from build123d import *

# Parameters (mm, degrees)
BOSS_EXTRUDE1_DEPTH     = 52
SHELL1_START            = 3
SHELL1_DEPTH            = 46
SKETCH2_R               = 4.5
BOSS_EXTRUDE2_DEPTH     = 52
SKETCH3_R               = 3.25
CUT_EXTRUDE1_DEPTH      = 49
SKETCH4_R               = 1.7
CUT_EXTRUDE2_DEPTH      = 91.166512631
CUT_EXTRUDE3_DEPTH      = 20
CUT_EXTRUDE3_DEPTH_BACK = 20
CUT_EXTRUDE4_DEPTH      = 3.5
SKETCH7_R               = 4
CUT_EXTRUDE5_DEPTH      = 3.5
SKETCH8_W               = 6
SKETCH8_H               = 37
BOSS_EXTRUDE3_DEPTH     = 8
SKETCH9_W               = 1.9
SKETCH9_H               = 33.6
CUT_EXTRUDE6_DEPTH      = 6
SKETCH10_R              = 3
BOSS_EXTRUDE4_DEPTH     = 8


# Read off the part's stored shape, not the designer's step: Shell1
with BuildPart() as part:
    # Sketch1 → Boss-Extrude1 (new body)
    with BuildSketch(Plane.XY):
        with BuildLine():
            Line((-45, -55), (45, -55))
            ThreePointArc((45, -55), (52.071067812, -52.071067812), (55, -45))
            Line((55, -45), (55, -10))
            ThreePointArc((55, -10), (52.071067812, -2.928932188), (45, 0))
            Line((45, 0), (-45, 0))
            ThreePointArc((-45, 0), (-52.071067812, -2.928932188), (-55, -10))
            Line((-55, -10), (-55, -45))
            ThreePointArc((-55, -45), (-52.071067812, -52.071067812), (-45, -55))
        make_face()
    extrude(amount=BOSS_EXTRUDE1_DEPTH)

    # Shell1 outline → Shell1 (cut)
    with BuildSketch(Plane.XY.offset(SHELL1_START)):
        with BuildLine():
            Line((45, -3), (45, 0))
            Line((45, 0), (-45, 0))
            Line((-45, 0), (-45, -3))
            ThreePointArc((-45, -3), (-49.949747468, -5.050252532), (-52, -10))
            Line((-52, -10), (-52, -45))
            ThreePointArc((-52, -45), (-49.949747468, -49.949747468), (-45, -52))
            Line((-45, -52), (45, -52))
            ThreePointArc((45, -52), (49.949747468, -49.949747468), (52, -45))
            Line((52, -45), (52, -10))
            ThreePointArc((52, -10), (49.949747468, -5.050252532), (45, -3))
        make_face()
    extrude(amount=SHELL1_DEPTH, mode=Mode.SUBTRACT)

    # Sketch2 → Boss-Extrude2 (add)
    with BuildSketch(Plane(origin=(0, 0, 0), x_dir=(1, 0, 0), z_dir=(0, 1, 0))):
        with Locations(Location((-40, -8, 0), (0, 0, 270))):
            Circle(SKETCH2_R)
        with Locations(Location((40, -8, 0), (0, 0, 270))):
            Circle(SKETCH2_R)
        with Locations(Location((-40, -40, 0), (0, 0, 270))):
            Circle(SKETCH2_R)
        with Locations(Location((40, -40, 0), (0, 0, 270))):
            Circle(SKETCH2_R)
    extrude(amount=-BOSS_EXTRUDE2_DEPTH)

    # Sketch3 → Cut-Extrude1 (cut)
    with BuildSketch(Plane.XZ.offset(55)):
        with Locations(Location((-40, 8, 0), (0, 0, 270))):
            Circle(SKETCH3_R)
        with Locations(Location((40, 8, 0), (0, 0, 270))):
            Circle(SKETCH3_R)
        with Locations(Location((-40, 40, 0), (0, 0, 270))):
            Circle(SKETCH3_R)
        with Locations(Location((40, 40, 0), (0, 0, 270))):
            Circle(SKETCH3_R)
    extrude(amount=-CUT_EXTRUDE1_DEPTH, mode=Mode.SUBTRACT)

    # Sketch4 → Cut-Extrude2 (cut, through all)
    with BuildSketch(Plane.XZ.offset(6)):
        with Locations(Location((-40, 8, 0), (0, 0, 270))):
            Circle(SKETCH4_R)
        with Locations(Location((40, 8, 0), (0, 0, 270))):
            Circle(SKETCH4_R)
        with Locations(Location((-40, 40, 0), (0, 0, 270))):
            Circle(SKETCH4_R)
        with Locations(Location((40, 40, 0), (0, 0, 270))):
            Circle(SKETCH4_R)
    extrude(amount=-CUT_EXTRUDE2_DEPTH, mode=Mode.SUBTRACT)

    # Sketch5 → Cut-Extrude3 (cut, two sides: drawn at the far end of the back side and taken through both)
    with BuildSketch(Plane.XY.offset(26).offset(-CUT_EXTRUDE3_DEPTH_BACK)):
        Polygon((-51, -14), (-51, -11.5), (-55.5, -16), (-55.5, -18.5), align=None)
        Polygon((51, -14), (51, -11.5), (55.5, -16), (55.5, -18.5), align=None)
        Polygon((-51, -20), (-51, -17.5), (-55.5, -22), (-55.5, -24.5), align=None)
        Polygon((51, -20), (51, -17.5), (55.5, -22), (55.5, -24.5), align=None)
        Polygon((-51, -26), (-51, -23.5), (-55.5, -28), (-55.5, -30.5), align=None)
        Polygon((51, -26), (51, -23.5), (55.5, -28), (55.5, -30.5), align=None)
        Polygon((-51, -32), (-51, -29.5), (-55.5, -34), (-55.5, -36.5), align=None)
        Polygon((51, -32), (51, -29.5), (55.5, -34), (55.5, -36.5), align=None)
        Polygon((-51, -38), (-51, -35.5), (-55.5, -40), (-55.5, -42.5), align=None)
        Polygon((51, -38), (51, -35.5), (55.5, -40), (55.5, -42.5), align=None)
    extrude(amount=CUT_EXTRUDE3_DEPTH + CUT_EXTRUDE3_DEPTH_BACK, mode=Mode.SUBTRACT)

    # Sketch6 → Cut-Extrude4 (cut)
    with BuildSketch(Plane.XZ.offset(55)):
        with BuildLine():
            Line((-34.5, 12), (-34.5, 40))
            ThreePointArc((-34.5, 40), (-33, 41.5), (-31.5, 40))
            Line((-31.5, 40), (-31.5, 12))
            ThreePointArc((-31.5, 12), (-33, 10.5), (-34.5, 12))
        make_face()
        with BuildLine():
            Line((-28.5, 12), (-28.5, 40))
            ThreePointArc((-28.5, 40), (-27, 41.5), (-25.5, 40))
            Line((-25.5, 40), (-25.5, 12))
            ThreePointArc((-25.5, 12), (-27, 10.5), (-28.5, 12))
        make_face()
        with BuildLine():
            Line((-22.5, 12), (-22.5, 40))
            ThreePointArc((-22.5, 40), (-21, 41.5), (-19.5, 40))
            Line((-19.5, 40), (-19.5, 12))
            ThreePointArc((-19.5, 12), (-21, 10.5), (-22.5, 12))
        make_face()
        with BuildLine():
            Line((-16.5, 12), (-16.5, 40))
            ThreePointArc((-16.5, 40), (-15, 41.5), (-13.5, 40))
            Line((-13.5, 40), (-13.5, 12))
            ThreePointArc((-13.5, 12), (-15, 10.5), (-16.5, 12))
        make_face()
        with BuildLine():
            Line((-10.5, 12), (-10.5, 40))
            ThreePointArc((-10.5, 40), (-9, 41.5), (-7.5, 40))
            Line((-7.5, 40), (-7.5, 12))
            ThreePointArc((-7.5, 12), (-9, 10.5), (-10.5, 12))
        make_face()
        with BuildLine():
            Line((-4.5, 12), (-4.5, 40))
            ThreePointArc((-4.5, 40), (-3, 41.5), (-1.5, 40))
            Line((-1.5, 40), (-1.5, 12))
            ThreePointArc((-1.5, 12), (-3, 10.5), (-4.5, 12))
        make_face()
        with BuildLine():
            Line((1.5, 12), (1.5, 40))
            ThreePointArc((1.5, 40), (3, 41.5), (4.5, 40))
            Line((4.5, 40), (4.5, 12))
            ThreePointArc((4.5, 12), (3, 10.5), (1.5, 12))
        make_face()
        with BuildLine():
            Line((7.5, 12), (7.5, 40))
            ThreePointArc((7.5, 40), (9, 41.5), (10.5, 40))
            Line((10.5, 40), (10.5, 12))
            ThreePointArc((10.5, 12), (9, 10.5), (7.5, 12))
        make_face()
        with BuildLine():
            Line((13.5, 12), (13.5, 40))
            ThreePointArc((13.5, 40), (15, 41.5), (16.5, 40))
            Line((16.5, 40), (16.5, 12))
            ThreePointArc((16.5, 12), (15, 10.5), (13.5, 12))
        make_face()
        with BuildLine():
            Line((19.5, 12), (19.5, 40))
            ThreePointArc((19.5, 40), (21, 41.5), (22.5, 40))
            Line((22.5, 40), (22.5, 12))
            ThreePointArc((22.5, 12), (21, 10.5), (19.5, 12))
        make_face()
    extrude(amount=-CUT_EXTRUDE4_DEPTH, mode=Mode.SUBTRACT)

    # Sketch7 → Cut-Extrude5 (cut)
    with BuildSketch(Plane(origin=(0, 0, 0), x_dir=(-1, 0, 0), z_dir=(0, 0, -1))):
        with Locations((30, -12)):
            Circle(SKETCH7_R)
        with Locations((-30, -12)):
            Circle(SKETCH7_R)
    extrude(amount=-CUT_EXTRUDE5_DEPTH, mode=Mode.SUBTRACT)

    # Sketch8 → Boss-Extrude3 (add)
    with BuildSketch(Plane(origin=(0, -52, 0), x_dir=(1, 0, 0), z_dir=(0, 1, 0))):
        with Locations((30, -26)):
            Rectangle(SKETCH8_W, SKETCH8_H)
    extrude(amount=BOSS_EXTRUDE3_DEPTH)

    # Sketch9 → Cut-Extrude6 (cut)
    with BuildSketch(Plane(origin=(0, -44, 0), x_dir=(1, 0, 0), z_dir=(0, 1, 0))):
        with Locations((30, -26)):
            Rectangle(SKETCH9_W, SKETCH9_H)
    extrude(amount=-CUT_EXTRUDE6_DEPTH, mode=Mode.SUBTRACT)

    # Sketch10 → Boss-Extrude4 (add)
    with BuildSketch(Plane(origin=(0, -52, 0), x_dir=(1, 0, 0), z_dir=(0, 1, 0))):
        with Locations(Location((-29, -13, 0), (0, 0, 55.426050329))):
            Circle(SKETCH10_R)
        with Locations(Location((-29, -39, 0), (0, 0, 80.405931773))):
            Circle(SKETCH10_R)
        with Locations(Location((13, -13, 0), (0, 0, 55.426050329))):
            Circle(SKETCH10_R)
        with Locations(Location((13, -39, 0), (0, 0, 80.405931773))):
            Circle(SKETCH10_R)
    extrude(amount=BOSS_EXTRUDE4_DEPTH)


solid = part.part
CAD build for the part. Positions are in the model's coordinates, mm. A direction names the side the tool comes from. Coordinates: 2 decimals unless noted, no trailing zeros. Write each loop counter-clockwise with the first axis right and the second up, starting at its lowest first coordinate (ties: lowest second). Pieces come first, ordered by that corner, then holes. Notation, with made-up numbers: (-19.75, 44) - (31.25, 44) arc R25 ccw to (31.25, 58) - close; hole circle Ø5 at (-26, -20). An arc over 180 degrees is marked (long way). Use a Markdown table: item, result. Add a question column.
Item 1: Band-saw the part on A-A, the plane x = -15. Give the cut face in (y, z).
Item 2: Band-saw the part on B-B, the plane z = 31.5. Give the number of separate pieces and of enclosed holes in the cut face, and give its area (3 significant figures).
Item 3: 3-axis set-ups, long thin cutter, end or side, ignore diameter. For faces 1 (the face through (13, -44, 13)), 2 (the face through (-53.5, -38, 25.7)), 3 (the face through (-27, -53.5, 10.5)): which of +Z, -Z, +X, -X, +Y, -Y reach the whole face in a straight line?
Item 4: Flat gauge pins, fed straight in: pin 1 (7 mm diameter, centred on x = -39, z = 9, fed in from -Y); pin 2 (1.5 mm diameter, centred on y = -53.5, z = 31.5, fed in from +X); pin 3 (1.8 mm diameter, centred on x = -28.5, z = 38, fed in from +Y); pin 4 (1 mm diameter, centred on x = 32.5, y = -12, fed in from -Z). Where does each tip first touch, or does it go through?
Item 5: Drill centre lines: L1, parallel to Z at x = -4, y = -39; L2, parallel to Z at x = -38, y = -22; L3, parallel to X at y = -31.5, z = 40. Where is each one in solid material? Low to high. Write a range as from..to.
Item 6: Mould opens along X. For faces 4 (the face through (51.99, -52.15, 25.64)), 5 (the face through (33, -48, 26)), 6 (the face through (1, 0, 50)) say: pulls with the +X half, pulls with the -X half, needs draft (parallel to the pull), parting line crosses it, or undercut.
Item 7: Band-saw the part on C-C, the plane x = 47.5. Give the cut face in (y, z).
Numbers:
| question | item | result |
|---|---|---|
| 1 | outline | (-55, 0) - (0, 0) - (0, 3) - (-52, 3) - (-52, 10.5) - (-55, 10.5) - close; (-55, 41.5) - (-52, 41.5) - (-52, 49) - (0, 49) - (0, 52) - (-55, 52) - close |
| 2 | separate pieces | 21 |
| 2 | enclosed holes | 0 |
| 2 | area | 512 mm2 |
| 3 | face 1 | +Y |
| 3 | face 2 | none |
| 3 | face 3 | -Y |
| 4 | pin 1 | y = -55 |
| 4 | pin 2 | x = 51.32 |
| 4 | pin 3 | y = -44 |
| 4 | pin 4 | z = 49 |
| 5 | L1 | 0..3, 49..52 |
| 5 | L2 | 0..3, 3.97..5.44, 10.56..12.03, 35.97..37.44, 42.56..44.03, 49..52 |
| 5 | L3 | -55..-53, -44.5..-43.25, -36.75..-35.5, 35.5..36.75, 43.25..44.5, 53..55 |
| 6 | face 4 | pulls with the +X half |
| 6 | face 5 | undercut |
| 6 | face 6 | needs draft |
| 7 | outline | (-54.68, 0) - (-0.32, 0) - (-0.32, 52) - (-54.68, 52) - close; hole (-51.54, 3) - (-3.46, 3) - (-3.46, 49) - (-51.54, 49) - close |
